```python
from build123d import *

# Parameters (mm, degrees)
BUITENAFMETING_RECHTHOEK_W  = 130
BUITENAFMETING_RECHTHOEK_H  = 190
PLAAT_DEPTH                 = 4
TAND_HOR_W                  = 18.571428572
TAND_HOR_H                  = 4
TAND_BOVEN_DEPTH            = 231.252035822
TANDEN_PATROON_BOVEN_COUNT  = 3
TANDEN_PATROON_BOVEN_PITCH  = 37.142857143
TAND_VER_W                  = 4
TAND_VER_H                  = 27.142857143
TAND_LINKS_DEPTH            = 231.252035822
TANDEN_PATROON_LINKS_COUNT  = 3
TANDEN_PATROON_LINKS_PITCH  = 54.285714286
TAND_O_W                    = 18.571428572
TAND_O_H                    = 4
TAND_ONDER_DEPTH            = 231.252035822
TANDEN_PATROON_ONDER_COUNT  = 3
TANDEN_PATROON_ONDER_PITCH  = 37.142857143
TAND_R_W                    = 4
TAND_R_H                    = 27.142857143
TAND_RECHTS_DEPTH           = 231.252035822
TANDEN_PATROON_RECHTS_COUNT = 3
TANDEN_PATROON_RECHTS_PITCH = 54.285714286
SKETCH1_W                   = 130
SKETCH1_H                   = 40
BOSS_EXTRUDE1_DEPTH         = 70
FILLET1_R                   = 5
CUT_EXTRUDE1_DEPTH          = 70
SKETCH4_R                   = 8
CUT_EXTRUDE2_DEPTH          = 27
SKETCH5_W                   = 75
SKETCH5_H                   = 140
BOSS_EXTRUDE2_DEPTH         = 5
SKETCH6_W                   = 65
SKETCH6_H                   = 129
CUT_EXTRUDE3_DEPTH          = 30


with BuildPart() as part:
    # Buitenafmeting Rechthoek → Plaat (new body)
    with BuildSketch(Plane.XY):
        with Locations((65, 95)):
            Rectangle(BUITENAFMETING_RECHTHOEK_W, BUITENAFMETING_RECHTHOEK_H)
    extrude(amount=-PLAAT_DEPTH)

    # Tand Hor → Tand Boven (cut, through all)
    with BuildSketch(Plane.XY):
        with Locations((27.857142857, 188)):
            Rectangle(TAND_HOR_W, TAND_HOR_H)
    tand_boven = extrude(amount=-TAND_BOVEN_DEPTH, mode=Mode.SUBTRACT)

    # Tanden Patroon Boven: Tand Boven ×3
    with Locations(*[(i * TANDEN_PATROON_BOVEN_PITCH, 0, 0) for i in range(1, TANDEN_PATROON_BOVEN_COUNT)]):
        add(tand_boven, mode=Mode.SUBTRACT)

    # Tand Ver → Tand Links (cut, through all)
    with BuildSketch(Plane.XY):
        with Locations((2, 149.285714286)):
            Rectangle(TAND_VER_W, TAND_VER_H)
    tand_links = extrude(amount=-TAND_LINKS_DEPTH, mode=Mode.SUBTRACT)

    # Tanden Patroon Links: Tand Links ×3
    with Locations(*[(0, -i * TANDEN_PATROON_LINKS_PITCH, 0) for i in range(1, TANDEN_PATROON_LINKS_COUNT)]):
        add(tand_links, mode=Mode.SUBTRACT)

    # Tand O → Tand Onder (cut, through all)
    with BuildSketch(Plane.XY):
        with Locations((27.857142857, 2)):
            Rectangle(TAND_O_W, TAND_O_H)
    tand_onder = extrude(amount=-TAND_ONDER_DEPTH, mode=Mode.SUBTRACT)

    # Tanden Patroon Onder: Tand Onder ×3
    with Locations(*[(i * TANDEN_PATROON_ONDER_PITCH, 0, 0) for i in range(1, TANDEN_PATROON_ONDER_COUNT)]):
        add(tand_onder, mode=Mode.SUBTRACT)

    # Tand R → Tand Rechts (cut, through all)
    with BuildSketch(Plane.XY):
        with Locations((128, 149.285714286)):
            Rectangle(TAND_R_W, TAND_R_H)
    tand_rechts = extrude(amount=-TAND_RECHTS_DEPTH, mode=Mode.SUBTRACT)

    # Tanden Patroon Rechts: Tand Rechts ×3
    with Locations(*[(0, -i * TANDEN_PATROON_RECHTS_PITCH, 0) for i in range(1, TANDEN_PATROON_RECHTS_COUNT)]):
        add(tand_rechts, mode=Mode.SUBTRACT)

    # Sketch1 → Boss-Extrude1 (add)
    with BuildSketch(Plane.XY):
        with Locations((65, 20)):
            Rectangle(SKETCH1_W, SKETCH1_H)
    extrude(amount=BOSS_EXTRUDE1_DEPTH)

    # Fillet1
    # the kernel refuses this fillet: 5 mm, written as the material it takes off along each edge
    with BuildSketch(Plane(origin=(5, 35, 65), x_dir=(0, 1, 0), z_dir=(-1, 0, 0))) as fillet1_piece_1_section:
        Polygon((0, 0), (FILLET1_R * 1.02, 0), (FILLET1_R * 1.02, -FILLET1_R * 1.02), (0, -FILLET1_R * 1.02), align=None)
    fillet1_piece_1 = extrude(amount=FILLET1_R * 1.02, mode=Mode.PRIVATE)
    fillet1_piece_1 = fillet1_piece_1 - Plane(origin=(5, 35, 65), x_dir=(0, -0.7071067811865475, -0.7071067811865475), z_dir=(-1, 0, 0)) * Sphere(FILLET1_R, mode=Mode.PRIVATE)
    add(fillet1_piece_1, mode=Mode.SUBTRACT)
    with BuildSketch(Plane(origin=(125, 35, 65), x_dir=(0, 0, 1), z_dir=(0, 1, 0))) as fillet1_piece_2_section:
        Polygon((0, 0), (FILLET1_R * 1.02, 0), (FILLET1_R * 1.02, FILLET1_R * 1.02), (0, FILLET1_R * 1.02), align=None)
    fillet1_piece_2 = extrude(amount=FILLET1_R * 1.02, mode=Mode.PRIVATE)
    fillet1_piece_2 = fillet1_piece_2 - Plane(origin=(125, 35, 65), x_dir=(-0.7071067811865475, 0, -0.7071067811865475), z_dir=(0, 1, 0)) * Sphere(FILLET1_R, mode=Mode.PRIVATE)
    add(fillet1_piece_2, mode=Mode.SUBTRACT)
    with BuildSketch(Plane(origin=(0, 40, 0), x_dir=(0, -1, 0), z_dir=(0, 0, 1)), Plane(origin=(130, 40, 0), x_dir=(-1, 0, 0), z_dir=(0, 0, 1))) as fillet1_piece_3:
        with BuildLine():
            CenterArc((FILLET1_R, FILLET1_R), FILLET1_R, 180, 90)
            Line((0, FILLET1_R), (0, 0))
            Line((0, 0), (FILLET1_R, 0))
        make_face()
    extrude(amount=65, mode=Mode.SUBTRACT)
    with BuildSketch(Plane(origin=(0, 35, 70), x_dir=(0, 0, -1), z_dir=(0, -1, 0))) as fillet1_piece_4:
        with BuildLine():
            CenterArc((FILLET1_R, FILLET1_R), FILLET1_R, 180, 90)
            Line((0, FILLET1_R), (0, 0))
            Line((0, 0), (FILLET1_R, 0))
        make_face()
    extrude(amount=47.5, mode=Mode.SUBTRACT)
    with BuildSketch(Plane(origin=(130, -12.5, 70), x_dir=(-1, 0, 0), z_dir=(0, 1, 0))) as fillet1_piece_5:
        with BuildLine():
            CenterArc((FILLET1_R, -FILLET1_R), FILLET1_R, 90, 90)
            Line((0, -FILLET1_R), (0, 0))
            Line((0, 0), (FILLET1_R, 0))
        make_face()
    extrude(amount=47.5, mode=Mode.SUBTRACT)
    with BuildSketch(Plane(origin=(125, 40, 70), x_dir=(0, 0, -1), z_dir=(-1, 0, 0))) as fillet1_piece_6:
        with BuildLine():
            CenterArc((FILLET1_R, FILLET1_R), FILLET1_R, 180, 90)
            Line((0, FILLET1_R), (0, 0))
            Line((0, 0), (FILLET1_R, 0))
        make_face()
    extrude(amount=120, mode=Mode.SUBTRACT)

    # Sketch2 → Cut-Extrude1 (cut)
    with BuildSketch(Plane(origin=(0, 0, -4), x_dir=(-1, 0, 0), z_dir=(0, 0, -1))):
        Polygon((-92.857142857, 4), (-4, 4), (-4, 36), (-92.857142857, 36), (-126, 36), (-126, 4), align=None)
    extrude(amount=-CUT_EXTRUDE1_DEPTH, mode=Mode.SUBTRACT)

    # Sketch4 → Cut-Extrude2 (cut)
    with BuildSketch(Plane(origin=(0, 40, 0), x_dir=(1, 0, 0), z_dir=(0, 1, 0))):
        with Locations(Location((65, -35, 0), (0, 0, 270))):
            Circle(SKETCH4_R)
        with Locations(Location((100, -35, 0), (0, 0, 270))):
            Circle(SKETCH4_R)
        with Locations(Location((30, -35, 0), (0, 0, 270))):
            Circle(SKETCH4_R)
    extrude(amount=-CUT_EXTRUDE2_DEPTH, mode=Mode.SUBTRACT)

    # Sketch5 → Boss-Extrude2 (add)
    with BuildSketch(Plane.XY):
        with Locations((65, 113)):
            Rectangle(SKETCH5_W, SKETCH5_H)
    extrude(amount=BOSS_EXTRUDE2_DEPTH)

    # Sketch6 → Cut-Extrude3 (cut)
    with BuildSketch(Plane.XY.offset(5)):
        with Locations((65, 113)):
            Rectangle(SKETCH6_W, SKETCH6_H)
    extrude(amount=-CUT_EXTRUDE3_DEPTH, mode=Mode.SUBTRACT)


solid = part.part
```
Here's how the part is built. I have some questions about the finished solid (model axes, mm). A direction names the side the tool comes from. Give positions to 0.01 mm unless a question says otherwise; leave off trailing zeros. Write each loop counter-clockwise with the first axis right and the second up, starting at its lowest first coordinate (ties: lowest second). Pieces come first, ordered by that corner, then holes. Notation, with made-up numbers: (-25, 85.5) -> (32, 85.5) arc R21 ccw to (32, 91.5) -> close; hole circle Ø1 at (88, 38.5). An arc over 180 degrees is marked (long way). Write each question's results on one line, items separated by ' | '.
Item 1: Suppose I cut it at D-D on z = 25. Write out the boundary of the cut face in (x, y).
Output:
outline: (0, 0) -> (130, 0) -> (130, 35) arc R5 ccw to (125, 40) -> (5, 40) arc R5 ccw to (0, 35) -> close; hole (4, 4) -> (126, 4) -> (126, 36) -> (4, 36) -> close
Item 2: We'd pull the mould along X, two halves only. Please class faces 4 (the face through (32.5, 112, 1)), 5 (the face through (109, 114, 0)), 6 (the face through (0, 122, -2)): pulls with the +X half, pulls with the -X half, needs draft (parallel to the pull), parting line crosses it, or undercut.
Output:
face 4: undercut | face 5: needs draft | face 6: pulls with the -X half
Item 3: Suppose I cut it at B-B on z = 35. Write out the boundary of the cut face in (x, y).
Output:
outline: (0, 0) -> (130, 0) -> (130, 35) arc R5 ccw to (125, 40) -> (108, 40) -> (108, 36) -> (126, 36) -> (126, 4) -> (4, 4) -> (4, 36) -> (22, 36) -> (22, 40) -> (5, 40) arc R5 ccw to (0, 35) -> close; (38, 36) -> (57, 36) -> (57, 40) -> (38, 40) -> close; (73, 36) -> (92, 36) -> (92, 40) -> (73, 40) -> close
Item 4: If I drill on L1, parallel to Y at x = 23, z = 4; L2, parallel to X at y = 21.5, z = 56; L3, parallel to X at y = 37.9, z = 35, over which ranges is the centre line in solid material (lowest first)?
Output:
L1: y = 0 to 4, 36 to 40 | L2: x = 0 to 4, 126 to 130 | L3: x = 0.93 to 22, 38 to 57, 73 to 92, 108 to 129.07
Item 5: On a 3-axis mill with a long thin cutter (end or side, diameter ignored), from which of +Z, -Z, +X, -X, +Y, -Y can I reach the whole of each face in a straight line? I mean faces 1 (the face through (65, 177.5, 1)), 2 (the face through (128, 162.857, -2)), 3 (the face through (2, 135.714, -2)). Say none if no direction works.
Output:
face 1: +Z, -Z | face 2: +Z, -Z, +X | face 3: +Z, -Z, -X
Item 6: Suppose I cut it at C-C on x = 65. Write out the boundary of the cut face in (y, z), plus the area to 3 significant figures.
Output:
outline: (0, 0) -> (4, 0) -> (4, 66) -> (36, 66) -> (36, 43) -> (40, 43) -> (40, 65) arc R5 ccw to (35, 70) -> (0, 70) -> close; (36, -4) -> (48.5, -4) -> (48.5, 5) -> (43, 5) -> (43, 0) -> (40, 0) -> (40, 27) -> (36, 27) -> close; (177.5, -4) -> (186, -4) -> (186, 0) -> (183, 0) -> (183, 5) -> (177.5, 5) -> close | area: 758 mm^2
Item 7: Suppose I cut it at A-A on y = 124.5. Write out the boundary of the cut face in (x, z), plus the area to 3 significant figures.
Output:
outline: (0, -4) -> (32.5, -4) -> (32.5, 5) -> (27.5, 5) -> (27.5, 0) -> (0, 0) -> close; (97.5, -4) -> (130, -4) -> (130, 0) -> (102.5, 0) -> (102.5, 5) -> (97.5, 5) -> close | area: 310 mm^2
Item 8: For pin 1 Ø1.5 at (x, z) = (56.5, 1.5) entering from -Y; pin 2 Ø1 at (x, z) = (106.5, 39.5) entering from +Y; pin 3 Ø2 at (x, y) = (67.5, 1) entering from -Z; pin 4 Ø2 at (x, z) = (27, -3) entering from +Y, each with a flat end and sliding along its axis, tell me the tip position at first contact or that it passes through.
Output:
pin 1: stops at y = 0 | pin 2: stops at y = 40 | pin 3: stops at z = 0 | pin 4: stops at y = 186
